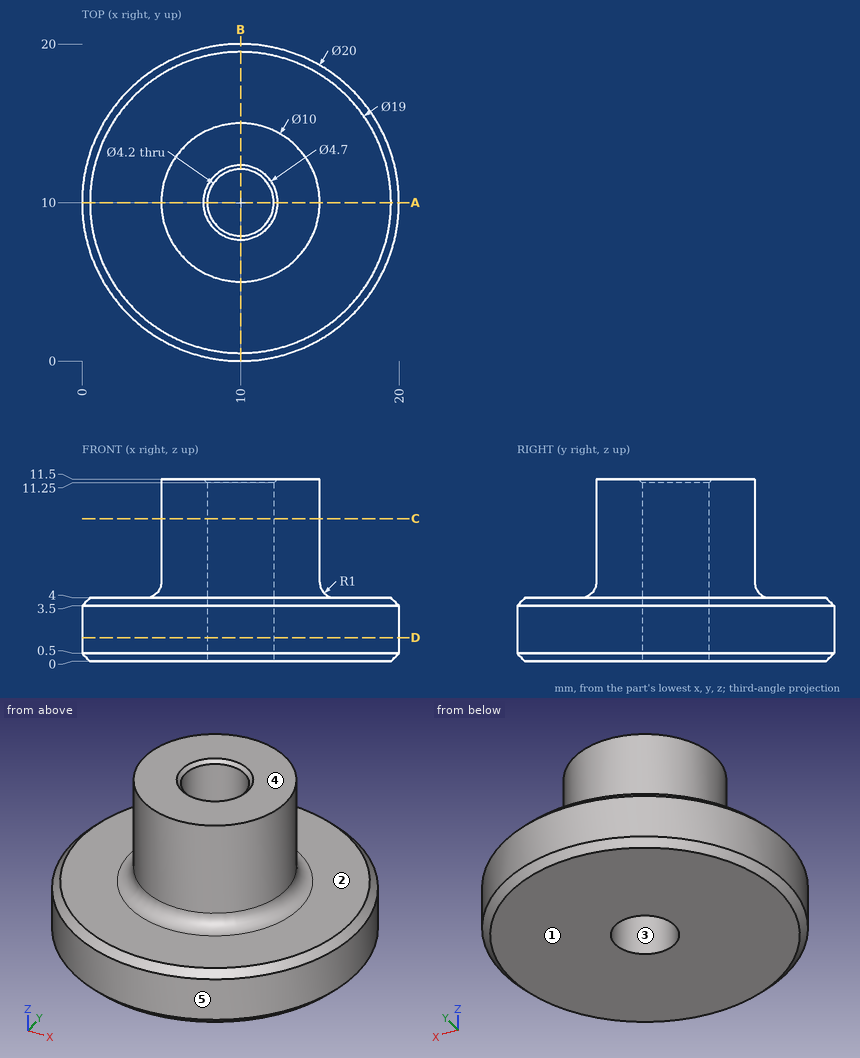
Can you work these out from the drawing? Everything is in mm from the part's minimum corner. A direction names the side the tool comes from. Round coordinates to 2 decimals unless told otherwise and drop trailing zeros. Write each loop counter-clockwise with the first axis right and the second up, starting at its lowest first coordinate (ties: lowest second). Pieces come first, ordered by that corner, then holes. Notation, with made-up numbers: (29.5, 18.5) - (87.5, 18.5) arc R28 ccw to (87.5, 42.5) - close; hole circle Ø2 at (-33.5, 61.25). An arc over 180 degrees is marked (long way). Use a Markdown table: item, result.
Q1. For pin 1 (3 mm diameter, centred on x = 16, z = 4, fed in from +Y); pin 2 (3 mm diameter, centred on x = 18, z = 7.5, fed in from +Y); pin 3 (3 mm diameter, centred on x = 2.5, y = 4, fed in from -Z); pin 4 (3 mm diameter, centred on x = 17, y = 16, fed in from +Z), each with a flat end and sliding along its axis, tell me the tip position at first contact or that it passes through.
Output values:
| item | result |
|---|---|
| pin 1 | y = 18.89 |
| pin 2 | through |
| pin 3 | z = 0 |
| pin 4 | z = 4 |
Q2. Please list where these lines run through material, in increasing order: L1, parallel to Y at x = 10, z = 5.5; L2, parallel to Y at x = 9.5, z = 9.75; L3, parallel to Z at x = 17, y = 15.5.
Output values:
| item | result |
|---|---|
| L1 | 5 to 7.9, 12.1 to 15 |
| L2 | 5.03 to 7.96, 12.04 to 14.97 |
| L3 | 0 to 4 |
Q3. For the marked faces 1 and 2, which set-ups out of +Z, -Z, +X, -X, +Y, -Y let a thin tool reach every point of the face, with its end or its side?
Output values:
| item | result |
|---|---|
| face 1 | -Z, +X, -X, +Y, -Y |
| face 2 | +Z |
Q4. I want a section at C-C (z = 9). List the corners of the cut face in (x, y) for me, plus the area to 3 significant figures.
Output values:
| item | result |
|---|---|
| outline | circle Ø10 at (10, 10); hole circle Ø4.2 at (10, 10) |
| area | 64.7 mm2 |
Q5. I want a section at D-D (z = 1.5). List the corners of the cut face in (x, y) for me.
Output values:
| item | result |
|---|---|
| outline | circle Ø20 at (10, 10); hole circle Ø4.2 at (10, 10) |
Q6. I want a section at A-A (y = 10). List the corners of the cut face in (x, z) for me, plus the area to 3 significant figures.
Output values:
| item | result |
|---|---|
| outline | (0, 0.5) - (0.5, 0) - (7.9, 0) - (7.9, 11.25) - (7.65, 11.5) - (5, 11.5) - (5, 5) arc R1 cw to (4, 4) - (0.5, 4) - (0, 3.5) - close; (12.1, 0) - (19.5, 0) - (20, 0.5) - (20, 3.5) - (19.5, 4) - (16, 4) arc R1 cw to (15, 5) - (15, 11.5) - (12.35, 11.5) - (12.1, 11.25) - close |
| area | 107 mm2 |
Q7. Thinking about a two-plate mould opening in X: for the marked faces 3, 4 and 5, which applies, released by +X, released by -X, zero draft, split by the parting line, or undercut?
Output values:
| item | result |
|---|---|
| face 3 | undercut |
| face 4 | zero draft |
| face 5 | split by the parting line |
